```python
from build123d import *

# Parameters (mm, degrees)
REVOLVE1_ANGLE = 270


with BuildPart() as part:
    # Sketch1 → Revolve1 (revolve)
    with BuildSketch(Plane.XY):
        Polygon((-50, -25), (-50.300177152, 2.198343583), (-16.300177152, 15), (0, 15), (0, 25), (20, 25), (20, 7.5), (50, 7.5), (50, -25), align=None)
    revolve(axis=Axis((50, -25, 0), (-1, 0, 0)), revolution_arc=REVOLVE1_ANGLE)

    # Sketch2 → Cut-Revolve1 (revolve, cut)
    with BuildSketch(Plane.XY):
        Polygon((-50.187622145, -8), (-16.203429147, -8), (-16.203429147, -13), (9.780588509, -13), (50, -2.223241171), (50, -25), (-50.300177152, -25), align=None)
    revolve(axis=Axis((50, -25, 0), (-1, 0, 0)), mode=Mode.SUBTRACT)


solid = part.part
```
Can you work these out from the model? Positions are in its coordinate system, mm. A direction names the side the tool comes from. Coordinates: 2 decimals unless noted, no trailing zeros. Loops run counter-clockwise (first coordinate to the right, second up) from the corner with the lowest first, then second, coordinate; pieces in that order, holes last.
1) I need wall thicknesses on probe 1 along Z at (x, y) = (43.5, -30); probe 2 along X at (y, z) = (17, -24); probe 3 along Z at (x, y) = (-2, -26.5). Which ranges of each line are inside material? Lowest first, please.
2) Thinking about a two-plate mould opening in Y: for faces 1 (the cylindrical face through (10.14, -59.17, -36.5)), 2 (the flat face through (1, 2, 0)), 3 (the cylindrical face through (-3.03, -33.2, -8.76)), which applies, pulls with the +Y half, pulls with the -Y half, needs draft (parallel to the pull), parting line crosses it, or undercut?
3) For pin 1 (19 mm diameter, centred on x = -5.5, y = 8, fed in from +Z); pin 2 (1.5 mm diameter, centred on x = -39, z = 26.5, fed in from -Y); pin 3 (21.5 mm diameter, centred on y = -25, z = 0, fed in from -X); pin 4 (4 mm diameter, centred on x = 21.5, z = -31, fed in from -Y), each with a flat end and sliding along its axis, tell me the tip position at first contact or that it passes through.
4) Imagine slicing it at B-B on x = 42. List the corners of the cut face in (y, z) for me.
5) Imagine slicing it at A-A on x = -5.5. List the corners of the cut face in (y, z) for me, plus the area to 3 significant figures.
6) Which directions (+Z, -Z, +X, -X, +Y, -Y) give clear straight access to the entire face, cutting with the end or side of a thin tool? Please do faces 4 (the flat face through (50, -42, -17)), 5 (the flat face through (1, -25, 27)), 6 (the flat face through (20, -59, -1)), 7 (the cylindrical face through (-32.96, -36.62, -12.41)).
Completed:
1. probe 1: z = -32.11 to -20.43, 20.43 to 32.11
1. probe 2: x = 0 to 20
1. probe 3: z = -39.97 to -11.91, 11.91 to 39.97
2. face 1: parting line crosses it
2. face 2: needs draft
2. face 3: undercut
3. pin 1: stops at z = 0
3. pin 2: stops at y = -43.17
3. pin 3: passes through
3. pin 4: stops at y = -65.24
4. outline: (-25, 20.63) - (-25, 32.5) arc R32.5 ccw (long way) to (7.5, 0) - (-4.37, 0) arc R20.63 cw (long way) to start
5. outline: (-25, 12) - (-25, 40) arc R40 ccw (long way) to (15, 0) - (-13, 0) arc R12 cw (long way) to start
5. area: 3,430 mm2
6. face 4: +Z, -Z, +X, +Y, -Y
6. face 5: +Z, +X, -X, +Y
6. face 6: +X
6. face 7: -X
